Input: part model. Units: mm. Frame: model coordinates. Give positions to 0.01 mm unless a question says otherwise; leave off trailing zeros. Loops run counter-clockwise (first coordinate to the right, second up) from the corner with the lowest first, then second, coordinate; pieces in that order, holes last. Notation, with made-up numbers: (63, 51.25) -> (104, 51.25) arc R10 cw to (104, 63.25) -> close; hole circle Ø1 at (-19.75, 81.5). An arc over 180 degrees is marked (long way). One line per question, with ' | ' between items.
from build123d import *

# Parameters (mm, degrees)
PATTERN_CIRCULAR_1_OUTLINE_R     = 1.5
PATTERN_CIRCULAR_1_DEPTH         = 5
PATTERN_START                    = 3
PATTERN_CIRCULAR_1_2_OUTLINE_R   = 2
PATTERN_CIRCULAR_1_2_OUTLINE_R_2 = 1.5
PATTERN_CIRCULAR_1_2_DEPTH       = 2


# Read off the part's stored shape, not the designer's step: Круговой массив1
with BuildPart() as part:
    # Эскиз1 → Повернуть1 (revolve)
    with BuildSketch(Plane(origin=(0, 0, 0), x_dir=(0, 0, -1), z_dir=(1, 0, 0))):
        with BuildLine():
            Line((0, 0), (30, 0))
            Line((30, 0), (30, 4))
            ThreePointArc((30, 4), (29.707106781, 4.707106781), (29, 5))
            Line((29, 5), (0, 5))
            Line((0, 5), (0, 0))
        make_face()
    revolve(axis=Axis((0, 0, 0), (0, 1, 0)))

    # Эскиз2 → Вырез-Повернуть1 (revolve, cut)
    with BuildSketch(Plane(origin=(0, 0, 0), x_dir=(0, 0, -1), z_dir=(1, 0, 0))):
        Polygon((-25, 0), (-23.5, 0), (-23.5, 3), (-23, 3), (-23, 5), (-25, 5), align=None)
    revolve(axis=Axis((0, 0, 25), (0, 1, 0)), mode=Mode.SUBTRACT)

    # Круговой массив1 outline → Круговой массив1 (cut)
    with BuildSketch(Plane(origin=(0, 0, 0), x_dir=(1, 0, 0), z_dir=(0, 1, 0))):
        with Locations((-21.650635095, -12.5)):
            Circle(PATTERN_CIRCULAR_1_OUTLINE_R)
        with Locations((-21.650635095, 12.5)):
            Circle(PATTERN_CIRCULAR_1_OUTLINE_R)
        with Locations((0, 25)):
            Circle(PATTERN_CIRCULAR_1_OUTLINE_R)
        with Locations((21.650635095, 12.5)):
            Circle(PATTERN_CIRCULAR_1_OUTLINE_R)
        with Locations((21.650635095, -12.5)):
            Circle(PATTERN_CIRCULAR_1_OUTLINE_R)
    extrude(amount=PATTERN_CIRCULAR_1_DEPTH, mode=Mode.SUBTRACT)

    # Pattern Circular 1 2 outline → Pattern Circular 1 2 (cut)
    # profile 1 of 5: a face of its own
    with BuildSketch(Plane(origin=(0, 0, 0), x_dir=(1, 0, 0), z_dir=(0, 1, 0)).offset(PATTERN_START)):
        with Locations((-21.650635095, -12.5)):
            Circle(PATTERN_CIRCULAR_1_2_OUTLINE_R)
        with Locations((-21.650635095, -12.5)):
            Circle(PATTERN_CIRCULAR_1_2_OUTLINE_R_2, mode=Mode.SUBTRACT)
    # profile 2 of 5: a face of its own
    with BuildSketch(Plane(origin=(0, 0, 0), x_dir=(1, 0, 0), z_dir=(0, 1, 0)).offset(PATTERN_START)):
        with Locations((-21.650635095, 12.5)):
            Circle(PATTERN_CIRCULAR_1_2_OUTLINE_R)
        with Locations((-21.650635095, 12.5)):
            Circle(PATTERN_CIRCULAR_1_2_OUTLINE_R_2, mode=Mode.SUBTRACT)
    # profile 3 of 5: a face of its own
    with BuildSketch(Plane(origin=(0, 0, 0), x_dir=(1, 0, 0), z_dir=(0, 1, 0)).offset(PATTERN_START)):
        with Locations((0, 25)):
            Circle(PATTERN_CIRCULAR_1_2_OUTLINE_R)
        with Locations((0, 25)):
            Circle(PATTERN_CIRCULAR_1_2_OUTLINE_R_2, mode=Mode.SUBTRACT)
    # profile 4 of 5: a face of its own
    with BuildSketch(Plane(origin=(0, 0, 0), x_dir=(1, 0, 0), z_dir=(0, 1, 0)).offset(PATTERN_START)):
        with Locations((21.650635095, 12.5)):
            Circle(PATTERN_CIRCULAR_1_2_OUTLINE_R)
        with Locations((21.650635095, 12.5)):
            Circle(PATTERN_CIRCULAR_1_2_OUTLINE_R_2, mode=Mode.SUBTRACT)
    # profile 5 of 5: a face of its own
    with BuildSketch(Plane(origin=(0, 0, 0), x_dir=(1, 0, 0), z_dir=(0, 1, 0)).offset(PATTERN_START)):
        with Locations((21.650635095, -12.5)):
            Circle(PATTERN_CIRCULAR_1_2_OUTLINE_R)
        with Locations((21.650635095, -12.5)):
            Circle(PATTERN_CIRCULAR_1_2_OUTLINE_R_2, mode=Mode.SUBTRACT)
    extrude(amount=PATTERN_CIRCULAR_1_2_DEPTH, mode=Mode.SUBTRACT)


solid = part.part
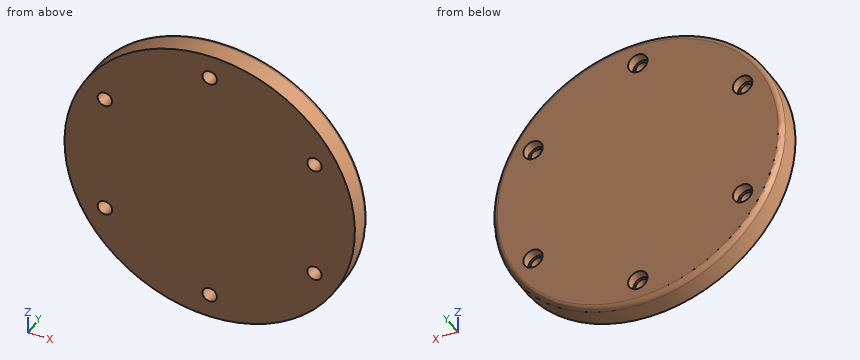
1. Pin query (flat end, axial travel): P1, Ø1.5, axis at y = 3.5, z = 10.5, coming from the +X side; P2, Ø1, axis at y = 4.5, z = 21, coming from the +X side; P3, Ø1.5, axis at y = 3.5, z = 5, coming from the -X side. Return the tip coordinate at first contact, or that it passes through.
Determined:
P1: stops at x = 28.37 | P2: stops at x = 21.8 | P3: stops at x = -29.7
2. Section query B-B (z = 12.5). Count the separate pieces of the cut face and the enclosed holes in it, then the cut area to 3 significant figures.
Determined:
separate pieces: 3 | enclosed holes: 0 | area: 238 mm2
3. Ray query, line 1 along Z through (x, y) = (0, 0.95); line 2 along Z through (x, y) = (0, 3.9); line 3 along X through (y, z) = (1.9, 12.5). Return the intervals inside material, ascending. Write a range as from..to.
Determined:
line 1: z = -30..-26.5, -23.5..23.5, 26.5..30 | line 2: z = -30..-27, -23..23, 27..30 | line 3: x = -27.27..-23.15, -20.15..20.15, 23.15..27.27
4. Section query A-A (x = 0). Output: boundary loops of the cut face in (y, z), then the cut area to 3 significant figures.
Determined:
outline: (0, -30) -> (4, -30) arc R1 ccw to (5, -29) -> (5, -27) -> (3, -27) -> (3, -26.5) -> (0, -26.5) -> close; (0, -23.5) -> (3, -23.5) -> (3, -23) -> (5, -23) -> (5, 23) -> (3, 23) -> (3, 23.5) -> (0, 23.5) -> close; (0, 26.5) -> (3, 26.5) -> (3, 27) -> (5, 27) -> (5, 29) arc R1 ccw to (4, 30) -> (0, 30) -> close | area: 266 mm2
